Source: three-view drawing plus pictorial views. Frame: mm from the lowest corner of the part. A direction names the side the tool comes from. Coordinates: 2 decimals unless noted, no trailing zeros. Order: outer loops, then holes, each group sorted by start corner. A loop starts at its lowest first (then second) coordinate and runs counter-clockwise, first axis right, second up. Notation, with made-up numbers: M 81.25,-26.5 L 93.25,-26.5 A30 ccw 93.25,5.5 Z; hole C 4,64 d7. An arc over 180 degrees is marked long. Use CSV: the item, a comma, the result in double quotes. Start each with the question number.
Q1. Section query A-A, the plane y = 6.35. Output: boundary loops of the cut face in (x, z) (3 decimals).
Q2. Section query B-B, the plane x = 16.75. Output: boundary loops of the cut face in (y, z), and give its area (3 significant figures).
Q3. First-contact query: P1, Ø3, axis at y = 11, z = 19.5, coming from the +X side (3 decimals); P2, Ø1, axis at y = 25.5, z = 40, coming from the -X side; P3, Ø7.5, axis at x = 13, z = 24.5, coming from the +Y side; P4, Ø5, axis at x = 19, y = 38, coming from the +Z side. Flat tips, straight axial feed; report the tip coordinate or a pass-through.
Q4. Access query for the marked faces 4, 5, 6, 7 and 8. Directions: +Z, -Z, +X, -X, +Y, -Y. A direction counts if a zero-diameter tool reaches every point of the face in a straight line with its end or side. Return the directions, or none.
Q5. Ray query, probe 1 along X at (y, z) = (22, 40) (3 decimals); probe 2 along Y at (x, z) = (1.75, 25); probe 3 along Y at (x, z) = (11.25, 9.5). Return the intervals inside material, ascending.
Q6. Section query D-D, the plane z = 10. Output: boundary loops of the cut face in (x, y) (1 decimal), and give its area (3 significant figures).
Q7. Section query C-C, the plane z = 4.5. Output: boundary loops of the cut face in (x, y) (3 decimals).
Q8. Mould query, pull axis Y, two halves, no side actions, for the marked faces 1, 2 and 3. Classes: +Y half, -Y half, draft (parallel to the pull), parting line (faces both ways), or undercut.
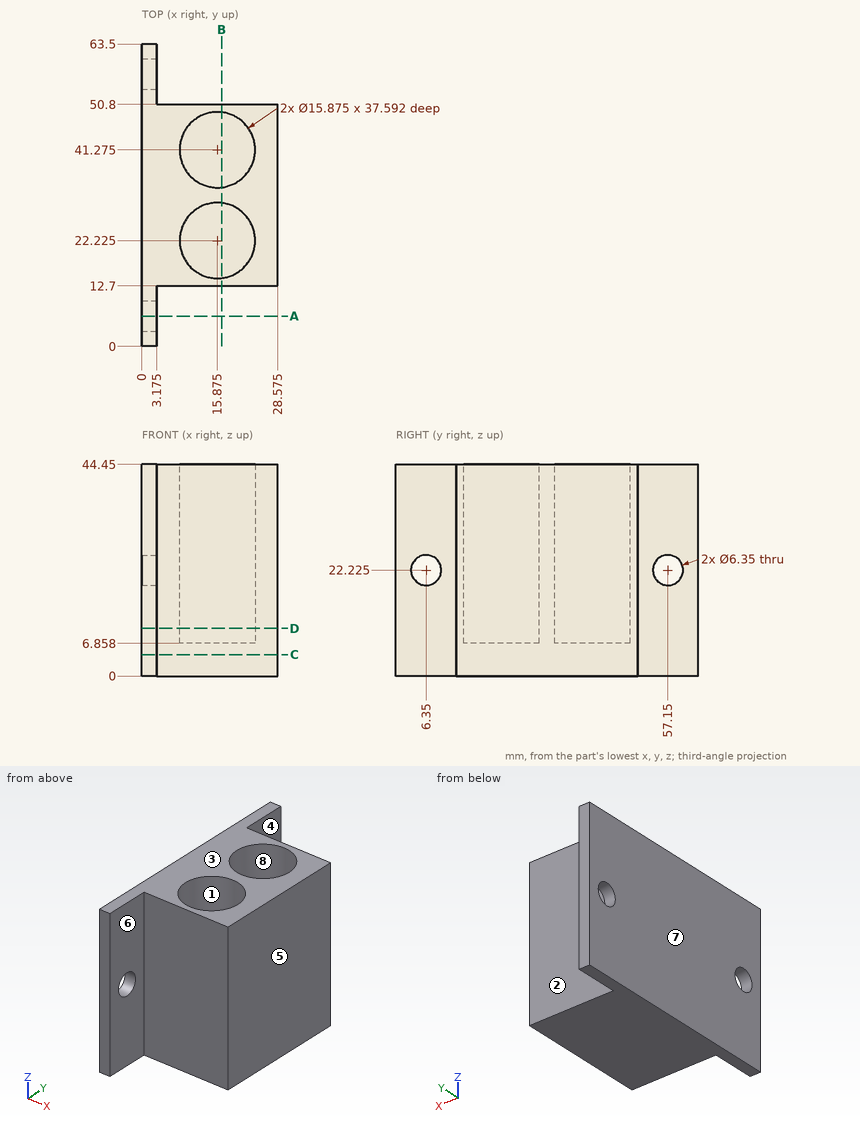
Responses:
1,outline,"M 0,0 L 3.175,0 L 3.175,19.05 L 0,19.05 Z; M 0,25.4 L 3.175,25.4 L 3.175,44.45 L 0,44.45 Z"
2,outline,"M 12.7,0 L 50.8,0 L 50.8,44.45 L 49.16,44.45 L 49.16,6.86 L 33.39,6.86 L 33.39,44.45 L 30.11,44.45 L 30.11,6.86 L 14.34,6.86 L 14.34,44.45 L 12.7,44.45 Z"
2,area,"507 mm²"
3,P1,"stops at x = 3.175"
3,P2,"stops at x = 0"
3,P3,"stops at y = 50.8"
3,P4,"stops at z = 6.86"
4,face 4,"+Z, -Z, +X, +Y"
4,face 5,"+Z, -Z, +X, +Y, -Y"
4,face 6,"+Z, -Z, +X, -Y"
4,face 7,"+Z, -Z, -X, +Y, -Y"
4,face 8,"+Z"
5,probe 1,"x = 0 to 7.941, 23.809 to 28.575"
5,probe 2,"y = 0 to 4.81, 7.89 to 55.61, 58.69 to 63.5"
5,probe 3,"y = 12.7 to 15.77, 28.68 to 34.82, 47.73 to 50.8"
6,outline,"M 0,0 L 3.2,0 L 3.2,12.7 L 28.6,12.7 L 28.6,50.8 L 3.2,50.8 L 3.2,63.5 L 0,63.5 Z; hole C 15.9,22.2 d15.9; hole C 15.9,41.3 d15.9"
6,area,"773 mm²"
7,outline,"M 0,0 L 3.175,0 L 3.175,12.7 L 28.575,12.7 L 28.575,50.8 L 3.175,50.8 L 3.175,63.5 L 0,63.5 Z"
8,face 1,"undercut"
8,face 2,"+Y half"
8,face 3,"draft"
